Autodesk Inventor part; units mm, degrees
ref_plane "YZ Plane" through (0, 0, 0) normal (1, 0, 0) x (0, 1, 0)
ref_plane "XZ Plane" through (0, 0, 0) normal (0, 1, 0) x (-1, 0, 0)
ref_plane "XY Plane" through (0, 0, 0) normal (0, 0, 1) x (1, 0, 0)
sketch "Sketch1" plane through (0, 0, 0) normal (0, 1, 0) x (-1, 0, 0)
  line L0 (0, 0) -> (-38.1, 0)
  line L1 (-38.1, 0) -> (-38.1, -101.6)
  line L2 (-38.1, -101.6) -> (0, -101.6)
  line L3 (0, -101.6) -> (0, 0)
  dimension "d0" = 38.1
  dimension "d1" = 101.6
extrude "Extrusion1" add sketch "Sketch1" along normal blind 3.175
sketch "Sketch3" plane through (0, 3.175, 0) normal (0, 1, 0) x (1, 0, 0)
  line L0 (31.75, 62.4332) -> (6.35, 62.4332)
  line L1 (6.35, 62.4332) -> (6.35, 37.0332)
  line L2 (6.35, 37.0332) -> (31.75, 37.0332)
  line L3 (31.75, 37.0332) -> (31.75, 62.4332)
  line L4 (38.1, 0) -> (38.1, 101.6)
  line L5 (38.1, 101.6) -> (0, 101.6)
  line L6 (28.575, 59.2582) -> (9.525, 59.2582)
  line L7 (9.525, 59.2582) -> (9.525, 40.2082)
  line L8 (9.525, 40.2082) -> (28.575, 40.2082)
  line L9 (28.575, 40.2082) -> (28.575, 59.2582)
  circle A0 centre (19.05, 49.7332) radius 2.54
  point P0 (0, 0)
  dimension "d8" = 25.4
  dimension "d9" = 25.4
  dimension "d10" = 6.35
  dimension "d11" = 39.1668
  dimension "d12" = 3.175
  dimension "d15" = 5.08
  dimension "d16" = 12.7
  dimension "d17" = 12.7
extrude "Extrusion3" add sketch "Sketch3" along normal blind 38.1 contours L3 L2 L1 L0
extrude "Extrusion5" cut sketch "Sketch3" against normal blind 3.175 contours A0
properties part number "mounting plate" material "ABS Plastic"
Can you work these out from the model? Positions are in its coordinate system, mm. A direction names the side the tool comes from. Give positions to 0.01 mm unless a question says otherwise; leave off trailing zeros. Loops run counter-clockwise (first coordinate to the right, second up) from the corner with the lowest first, then second, coordinate; pieces in that order, holes last. Notation, with made-up numbers: (85, 50.5) - (109, 50.5) arc R32 cw to (109, 83.5) - close; hole circle Ø4 at (79.25, -32). An arc over 180 degrees is marked (long way). Return JSON: item names as keys, results as strings.
1. We'd pull the mould along Z, two halves only. Please class faces 4 (the face through (21, 3.175, -52)), 5 (the face through (19, 2, 0)), 6 (the face through (38.1, 2, -50)): +Z half, -Z half, draft (parallel to the pull), parting line (faces both ways), or undercut.
Output values:
{"face 4": "undercut", "face 5": "+Z half", "face 6": "draft"}
2. I want a section at A-A on x = 19.05. Please give me the cut outline in (y, z) (3 decimals), and give its area (3 significant figures).
Output values:
{"outline": "(0, -101.6) - (3.175, -101.6) - (3.175, -62.433) - (41.275, -62.433) - (41.275, -59.258) - (3.175, -59.258) - (3.175, -52.273) - (0, -52.273) - close; (0, -47.193) - (3.175, -47.193) - (3.175, -40.208) - (41.275, -40.208) - (41.275, -37.033) - (3.175, -37.033) - (3.175, 0) - (0, 0) - close", "area": "548 mm²"}
3. For faces 1 (the face through (31.75, 22, -50)), 2 (the face through (9.525, 22, -50)), 3 (the face through (19, 22, -37.033)), which set-ups out of +Z, -Z, +X, -X, +Y, -Y let a thin tool reach every point of the face, with its end or its side?
Output values:
{"face 1": "+Z, -Z, +X, +Y", "face 2": "+Y", "face 3": "+Z, +X, -X, +Y"}
4. I'm going to push flat-ended pins straight in: pin 1 Ø8 at (x, z) = (32.5, -23.5) entering from +Y (3 decimals); pin 2 Ø5 at (y, z) = (22.5, -64.5) entering from -X; pin 3 Ø12.5 at (y, z) = (18, -52.5) entering from +X. Where does each tip first touch, or does it pass through?
Output values:
{"pin 1": "stops at y = 3.175", "pin 2": "stops at x = 6.35", "pin 3": "stops at x = 31.75"}
5. I want a section at B-B on y = 13.5. Please give me the cut outline in (x, z) (3 decimals), and give its area (3 significant figures).
Output values:
{"outline": "(6.35, -62.433) - (31.75, -62.433) - (31.75, -37.033) - (6.35, -37.033) - close; hole (9.525, -59.258) - (28.575, -59.258) - (28.575, -40.208) - (9.525, -40.208) - close", "area": "282 mm²"}
6. I want a section at D-D on x = 34. Please give me the cut outline in (y, z) (3 decimals), and give its area (3 significant figures).
Output values:
{"outline": "(0, -101.6) - (3.175, -101.6) - (3.175, 0) - (0, 0) - close", "area": "323 mm²"}
7. If I drill on line 1 (X direction, y = 33, z = -52.5) (3 decimals); line 2 (Z direction, x = 19.05, y = 0.8); line 3 (Z direction, x = 22, y = 8.5), over which ranges is the centre line in solid material (lowest first)?
Output values:
{"line 1": "x = 6.35 to 9.525, 28.575 to 31.75", "line 2": "z = -101.6 to -52.27, -47.19 to 0", "line 3": "z = -62.43 to -59.26, -40.21 to -37.03"}
8. I want a section at C-C on z = -90. Please give me the cut outline in (x, y) (3 decimals).
Output values:
{"outline": "(0, 0) - (38.1, 0) - (38.1, 3.175) - (0, 3.175) - close"}
